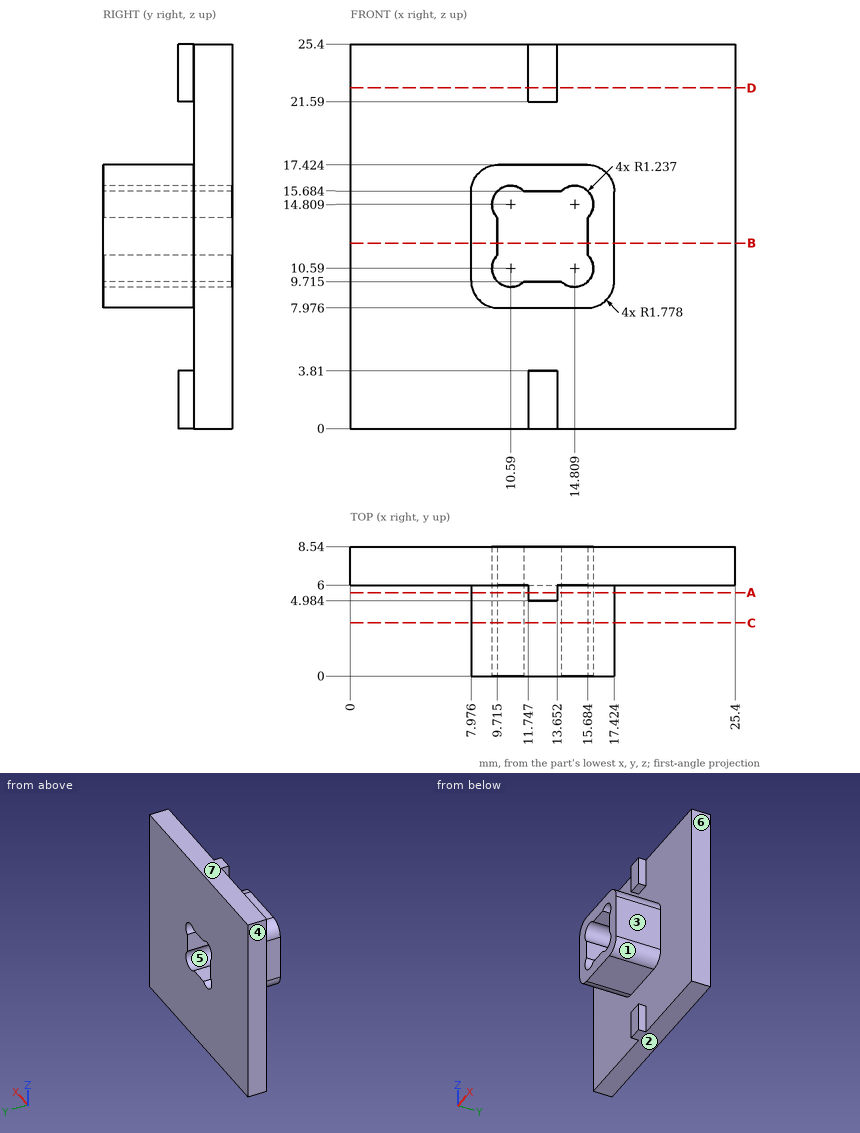
Drawing for the job (mm, zero at the part's lowest x, y, z). A direction names the side the tool comes from. Give positions to 0.01 mm unless a question says otherwise; leave off trailing zeros. Order: outer loops, then holes, each group sorted by start corner. A loop starts at its lowest first (then second) coordinate and runs counter-clockwise, first axis right, second up. Notation, with made-up numbers: M 11.5,-14 L 62.5,-14 A36 cw 62.5,25 Z; hole C 77,-12.75 d7. An arc over 180 degrees is marked long. Write item = value, one per line. Start each with the question number.
(1) Slice it at C-C on y = 3.5. Write the cut outline in (x, z) (1 decimal).
(2) Which spindle directions (+Z, -Z, +X, -X, +Y, -Y) get a long thin tool onto all of the face, cutting with end or side? Do the marked faces 1, 2 and 3. Say none if no direction does.
(3) Slice it at D-D on z = 22.5. Write the cut outline in (x, y) (1 decimal).
(4) Probe L1, parallel to X at y = 2, z = 13.5 (1 decimal); L2, parallel to Y at x = 5.25, z = 5; L3, parallel to X at y = 7.5, z = 10.5. List the from-to ranges inside material, lowest first. Write a range as [from, to].
(5) Two-plate mould, pull along X, no slides. Class the marked faces 4, 5, 6 and 7: released by +X, released by -X, zero draft, split by the parting line, or undercut.
(6) Pin check, flat tips, straight feed: pin 1 Ø1.2 at (y, z) = (3.5, 12) entering from +X; pin 2 Ø1.1 at (y, z) = (5.5, 24.5) entering from -X; pin 3 Ø2.5 at (x, y) = (13, 2.5) entering from +Z; pin 4 Ø2 at (x, z) = (13, 24) entering from -Y. Stop position of each tip, or through.
(7) Slice it at B-B on z = 12.25. Write the cut outline in (x, y) (1 decimal).
(8) Slice it at A-A on y = 5.5. Write the cut outline in (x, z) (1 decimal).
Responses:
q1.outline = M 8,9.8 A1.8 ccw 9.8,8 L 15.6,8 A1.8 ccw 17.4,9.8 L 17.4,15.6 A1.8 ccw 15.6,17.4 L 9.8,17.4 A1.8 ccw 8,15.6 Z; hole M 9.7,11.5 A1.2 ccw 11.5,9.7 L 13.9,9.7 A1.2 ccw 15.7,11.5 L 15.7,13.9 A1.2 ccw 13.9,15.7 L 11.5,15.7 A1.2 ccw 9.7,13.9 Z
q2.face_1 = -Z, +X, -Y
q2.face_2 = -Z, +X, -X, +Y, -Y
q2.face_3 = +Z, -Z, +X, -Y
q3.outline = M 0,6 L 11.7,6 L 11.7,5 L 13.7,5 L 13.7,6 L 25.4,6 L 25.4,8.5 L 0,8.5 Z
q4.L1 = [8, 9.7], [15.7, 17.4]
q4.L2 = [6, 8.54]
q4.L3 = [0, 9.36], [16.04, 25.4]
q5.face_4 = released by -X
q5.face_5 = undercut
q5.face_6 = released by +X
q5.face_7 = zero draft
q6.pin_1 = 17.42
q6.pin_2 = 0
q6.pin_3 = 17.42
q6.pin_4 = 4.98
q7.outline = M 0,6 L 8,6 L 8,0 L 9.7,0 L 9.7,8.5 L 0,8.5 Z; M 15.7,0 L 17.4,0 L 17.4,6 L 25.4,6 L 25.4,8.5 L 15.7,8.5 Z
q8.outline = M 8,9.8 A1.8 ccw 9.8,8 L 15.6,8 A1.8 ccw 17.4,9.8 L 17.4,15.6 A1.8 ccw 15.6,17.4 L 9.8,17.4 A1.8 ccw 8,15.6 Z; M 11.7,0 L 13.7,0 L 13.7,3.8 L 11.7,3.8 Z; M 11.7,21.6 L 13.7,21.6 L 13.7,25.4 L 11.7,25.4 Z; hole M 9.7,11.5 A1.2 ccw 11.5,9.7 L 13.9,9.7 A1.2 ccw 15.7,11.5 L 15.7,13.9 A1.2 ccw 13.9,15.7 L 11.5,15.7 A1.2 ccw 9.7,13.9 Z
